from build123d import *

# Parameters (mm, degrees)
SKETCH1_W           = 163.2
SKETCH1_H           = 73.6
BOSS_EXTRUDE1_DEPTH = 8.7
FILLET1_R           = 7
FILLET2_R           = 2
SKETCH2_R           = 1.5
BOSS_EXTRUDE2_DEPTH = 0.1
FILLET3_R           = 2
SKETCH3_W           = 40
SKETCH3_H           = 22
BOSS_EXTRUDE3_DEPTH = 1
FILLET4_R           = 4
CUT_EXTRUDE1_DEPTH  = 1
SKETCH5_R           = 5
SKETCH5_R_2         = 2.5
SKETCH5_R_3         = 2
BOSS_EXTRUDE4_DEPTH = 1
SKETCH6_R           = 4
SKETCH6_R_2         = 1.4
SKETCH6_R_3         = 1
BOSS_EXTRUDE5_DEPTH = 0.1


with BuildPart() as part:
    # Sketch1 → Boss-Extrude1 (new body)
    with BuildSketch(Plane(origin=(0, 0, 0), x_dir=(1, 0, 0), z_dir=(0, 1, 0))):
        Rectangle(SKETCH1_W, SKETCH1_H)
    extrude(amount=BOSS_EXTRUDE1_DEPTH)

    # Fillet1
    fillet1_edges = [part.edges().sort_by_distance(p)[0] for p in [
        (81.6, 4.35, 36.8),
        (-81.6, 4.35, 36.8),
        (-81.6, 4.35, -36.8),
        (81.6, 4.35, -36.8),
    ]]
    fillet(fillet1_edges, radius=FILLET1_R)

    # Fillet2
    fillet2_edges = [part.edges().sort_by_distance(p)[0] for p in [
        (81.6, 8.7, 0),
        (0, 8.7, 36.8),
        (0, 8.7, -36.8),
        (-81.6, 8.7, 0),
        (-79.549747468, 8.7, 34.749747468),
        (-79.549747468, 8.7, -34.749747468),
        (79.549747468, 8.7, -34.749747468),
        (79.549747468, 8.7, 34.749747468),
    ]]
    fillet(fillet2_edges, radius=FILLET2_R)

    # Sketch2 → Boss-Extrude2 (add)
    with BuildSketch(Plane(origin=(0, 8.7, 0), x_dir=(1, 0, 0), z_dir=(0, 1, 0))):
        with Locations(Location((-74.6, -27.8, 0), (0, 0, 90))):
            Circle(SKETCH2_R)
    extrude(amount=BOSS_EXTRUDE2_DEPTH)

    # Fillet3
    fillet3_edges = [part.edges().sort_by_distance(p)[0] for p in [
        (81.6, 0, 0),
        (0, 0, 36.8),
        (-81.6, 0, 0),
        (0, 0, -36.8),
        (-79.549747468, 0, 34.749747468),
        (-79.549747468, 0, -34.749747468),
        (79.549747468, 0, -34.749747468),
        (79.549747468, 0, 34.749747468),
    ]]
    fillet(fillet3_edges, radius=FILLET3_R)

    # Sketch3 → Boss-Extrude3 (add)
    with BuildSketch(Plane.XZ):
        with Locations((-54.6, -17.8)):
            Rectangle(SKETCH3_W, SKETCH3_H)
    extrude(amount=BOSS_EXTRUDE3_DEPTH)

    # Fillet4
    fillet4_edges = [part.edges().sort_by_distance(p)[0] for p in [
        (-74.6, -0.5, -6.8),
        (-74.6, -0.5, -28.8),
        (-34.6, -0.5, -28.8),
        (-34.6, -0.5, -6.8),
    ]]
    fillet(fillet4_edges, radius=FILLET4_R)

    # Sketch4 → Cut-Extrude1 (cut)
    with BuildSketch(Plane.XZ.offset(1)):
        with BuildLine():
            Line((-70.6, -27.8), (-38.6, -27.8))
            ThreePointArc((-38.6, -27.8), (-36.478679656, -26.921320344), (-35.6, -24.8))
            Line((-35.6, -24.8), (-35.6, -10.8))
            ThreePointArc((-35.6, -10.8), (-36.478679656, -8.678679656), (-38.6, -7.8))
            Line((-38.6, -7.8), (-70.6, -7.8))
            ThreePointArc((-70.6, -7.8), (-72.721320344, -8.678679656), (-73.6, -10.8))
            Line((-73.6, -10.8), (-73.6, -24.8))
            ThreePointArc((-73.6, -24.8), (-72.721320344, -26.921320344), (-70.6, -27.8))
        make_face()
    extrude(amount=-CUT_EXTRUDE1_DEPTH, mode=Mode.SUBTRACT)

    # Sketch5 → Boss-Extrude4 (add)
    with BuildSketch(Plane(origin=(0, 0, 0), x_dir=(-1, 0, 0), z_dir=(0, -1, 0))):
        with Locations(Location((66.6, 20.8, 0), (0, 0, 90))):
            Circle(SKETCH5_R)
        with Locations(Location((52.6, 20.8, 0), (0, 0, 90))):
            Circle(SKETCH5_R)
        with Locations(Location((40.6, 22.05, 0), (0, 0, 90))):
            Circle(SKETCH5_R_2)
        with Locations(Location((40.6, 13.55, 0), (0, 0, 90))):
            Circle(SKETCH5_R_2)
        with Locations(Location((59.6, 12.314718626, 0), (0, 0, 90))):
            Circle(SKETCH5_R_3)
    extrude(amount=BOSS_EXTRUDE4_DEPTH)

    # Sketch6 → Boss-Extrude5 (add)
    with BuildSketch(Plane.XZ.offset(1)):
        with Locations(Location((-66.6, -20.8, 0), (0, 0, 270))):
            Circle(SKETCH6_R)
        with Locations(Location((-52.6, -20.8, 0), (0, 0, 270))):
            Circle(SKETCH6_R)
        with Locations(Location((-40.6, -22.05, 0), (0, 0, 270))):
            Circle(SKETCH6_R_2)
        with Locations(Location((-40.6, -13.55, 0), (0, 0, 270))):
            Circle(SKETCH6_R_2)
        with Locations(Location((-59.6, -12.314718626, 0), (0, 0, 270))):
            Circle(SKETCH6_R_3)
    extrude(amount=BOSS_EXTRUDE5_DEPTH)


solid = part.part
The model under review builds one solid part; all positions refer to its coordinate system, in mm. A direction names the side the tool comes from. Give positions to 0.01 mm unless a question says otherwise; leave off trailing zeros. Order: outer loops, then holes, each group sorted by start corner. A loop starts at its lowest first (then second) coordinate and runs counter-clockwise, first axis right, second up. Notation, with made-up numbers: M -19.75,19 L -2.75,19 A9 cw -2.75,26 Z; hole C -3,55 d7. An arc over 180 degrees is marked long. Use one line per item in the form item = value. Start each with the question number.
Item 1: The part is to be moulded in two halves that separate along X. For faces 1 (the flat face through (-1, 4, -36.8)), 2 (the cylindrical face through (79.5, 4.4, 34.8)), 3 (the flat face through (-55, 0, -15)), 4 (the cylindrical face through (-73.459, -0.507, -27.597)), say which applies: pulls with the +X half, pulls with the -X half, needs draft (parallel to the pull), parting line crosses it, or undercut.
Item 2: We need section C-C on z = 12.5. Give the boundary of the cut face in (x, y), plus the area to 3 significant figures.
Item 3: We need section B-B on x = -52.6. Give the boundary of the cut face in (y, z), plus the area to 3 significant figures.
Item 4: To check wall thickness, follow line 1 along Y through (x, z) = (-28.5, 13); line 2 along Z through (x, y) = (1, 8.25); line 3 along X through (y, z) = (8, 2.5). State the ranges of each line that lie inside material, in increasing order. Write a range as from..to.
Item 5: We need section A-A on z = 27.8. Give the boundary of the cut face in (x, y), plus the area to 3 significant figures.
Item 6: We need section D-D on x = 2. Give the boundary of the cut face in (y, z).
Item 7: Insertion check: pin 1 Ø8 at (x, z) = (52, -4.5) entering from -Y; pin 2 Ø0.8 at (x, y) = (-60.5, -0.5) entering from -Z; pin 3 Ø0.5 at (x, y) = (-52.5, -0.5) entering from +Z. Each pin has a flat end and moves straight along its axis. Give the tip position at first contact, or say it passes through.
Item 8: For faces 5 (the cylindrical face through (-35.741, -0.507, -27.597)), 6 (the cylindrical face through (-72.7, -0.51, -8.66)), 7 (the flat face through (-75, 8.8, 28)), list the 3-axis set-ups (+Z, -Z, +X, -X, +Y, -Y) from which the entire face can be reached by the end or side of a thin tool; tool diameter is ignored.
Completed:
q1.face_1 = needs draft
q1.face_2 = pulls with the +X half
q1.face_3 = undercut
q1.face_4 = pulls with the -X half
q2.outline = M -81.6,2 A2 ccw -79.6,0 L 79.6,0 A2 ccw 81.6,2 L 81.6,6.7 A2 ccw 79.6,8.7 L -79.6,8.7 A2 ccw -81.6,6.7 Z
q2.area = 1,420 mm²
q3.outline = M -1.1,-24.8 L -1,-24.8 L -1,-25.8 L 0,-25.8 L 0,-27.8 L -1,-27.8 L -1,-28.8 L 0,-28.8 L 0,-34.8 A2 ccw 2,-36.8 L 6.7,-36.8 A2 ccw 8.7,-34.8 L 8.7,34.8 A2 ccw 6.7,36.8 L 2,36.8 A2 ccw 0,34.8 L 0,-6.8 L -1,-6.8 L -1,-7.8 L 0,-7.8 L 0,-15.8 L -1,-15.8 L -1,-16.8 L -1.1,-16.8 Z
q3.area = 650 mm²
q4.line_1 = 0..8.7
q4.line_2 = -36.06..36.06
q4.line_3 = -81.12..81.12
q5.outline = M -81.6,2 A2 ccw -79.6,0 L 79.6,0 A2 ccw 81.6,2 L 81.6,6.7 A2 ccw 79.6,8.7 L -73.1,8.7 L -73.1,8.8 L -76.1,8.8 L -76.1,8.7 L -79.6,8.7 A2 ccw -81.6,6.7 Z
q5.area = 1,420 mm²
q6.outline = M 0,-34.8 A2 ccw 2,-36.8 L 6.7,-36.8 A2 ccw 8.7,-34.8 L 8.7,34.8 A2 ccw 6.7,36.8 L 2,36.8 A2 ccw 0,34.8 Z
q7.pin_1 = 0
q7.pin_2 = -28.8
q7.pin_3 = -6.8
q8.face_5 = -Z, +X, -Y
q8.face_6 = -Y
q8.face_7 = +Z, -Z, +X, -X, +Y
